Input: dimensioned drawing with shaded views. Units: mm. Origin: part minimum x, y, z. Coordinates: 2 decimals unless noted, no trailing zeros. Loops run counter-clockwise (first coordinate to the right, second up) from the corner with the lowest first, then second, coordinate; pieces in that order, holes last.
(1) Line query: L1, parallel to Y at x = 38.1, z = 12.5; L2, parallel to Y at x = 69.85, z = 5.5 (3 decimals); L3, parallel to X at y = 4.5, z = 4. Output: solid intervals per line, ascending.
(2) Section C-C, the plane z = 2.5. Give the number of separate pieces and of enclosed holes in the cut face, then the cut area to 3 significant figures.
(3) Section B-B, the plane y = 12.7. Return loops of the section in (x, z).
(4) Section A-A, the plane x = 6.35. Return loops of the section in (y, z) (3 decimals).
(5) Section D-D, the plane x = 25.4. Return loops of the section in (y, z).
(6) Mould query, pull axis X, two halves, no side actions, for the marked faces 1, 2 and 3. Classes: released by +X, released by -X, zero draft, split by the parting line, or undercut.
(7) Contact query for a flat-ended pin moving along its axis: P1, Ø7.5, axis at x = 38.1, y = 12.7, coming from the +Z side. Output: stop coordinate, or through.
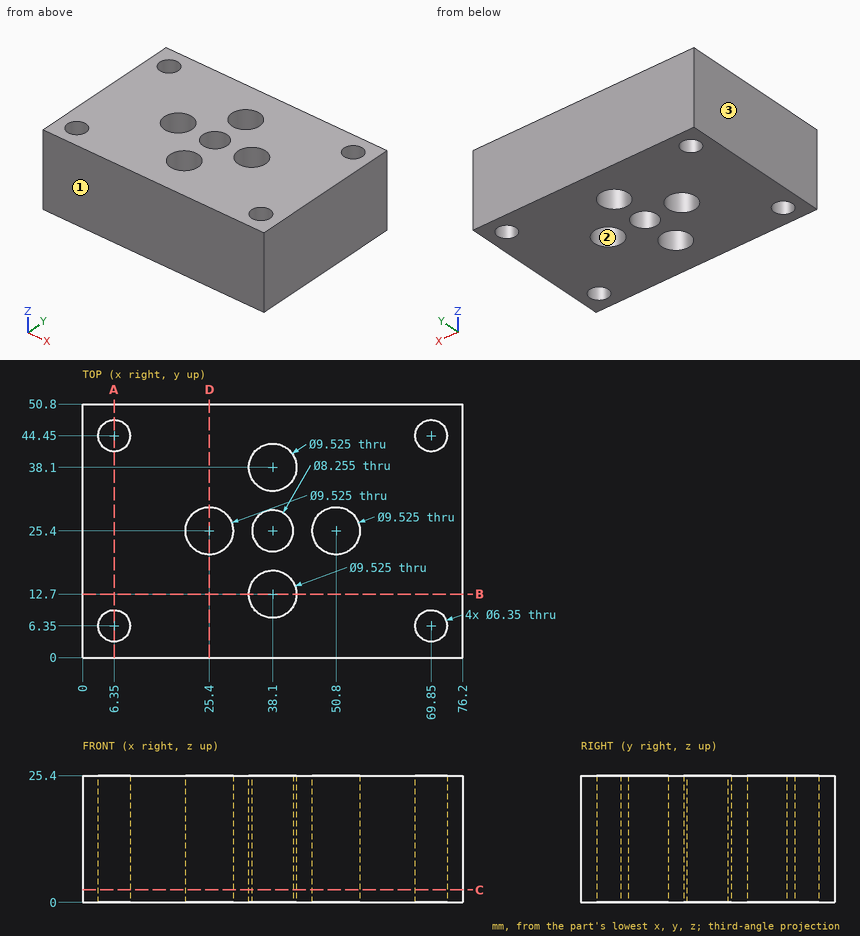
Report:
1. L1: y = 0 to 7.94, 17.46 to 21.27, 29.53 to 33.34, 42.86 to 50.8
1. L2: y = 0 to 3.175, 9.525 to 41.275, 47.625 to 50.8
1. L3: x = 0 to 3.77, 8.93 to 67.27, 72.43 to 76.2
2. separate pieces: 1
2. enclosed holes: 9
2. area: 3,410 mm2
3. outline: (0, 0) - (33.34, 0) - (33.34, 25.4) - (0, 25.4) - close; (42.86, 0) - (76.2, 0) - (76.2, 25.4) - (42.86, 25.4) - close
4. outline: (0, 0) - (3.175, 0) - (3.175, 25.4) - (0, 25.4) - close; (9.525, 0) - (41.275, 0) - (41.275, 25.4) - (9.525, 25.4) - close; (47.625, 0) - (50.8, 0) - (50.8, 25.4) - (47.625, 25.4) - close
5. outline: (0, 0) - (20.64, 0) - (20.64, 25.4) - (0, 25.4) - close; (30.16, 0) - (50.8, 0) - (50.8, 25.4) - (30.16, 25.4) - close
6. face 1: zero draft
6. face 2: undercut
6. face 3: released by -X
7. P1: passes through
